from build123d import *

# Parameters (mm, degrees)
SKETCH_1_W          = 24
SKETCH_1_H          = 70
EXTRUDE_1_DEPTH     = 30
SKETCH_2_R          = 7.55
CUT_EXTRUDE_1_DEPTH = 71.806439045
SKETCH_3_W          = 25
SKETCH_3_H          = 10
CUT_EXTRUDE_2_DEPTH = 71.806439045
SKETCH_4_W          = 24
SKETCH_4_H          = 9.317438099
EXTRUDE_2_DEPTH     = 5
SKETCH_5_R          = 1.55
CUT_EXTRUDE_3_DEPTH = 31
FILLET_1_R          = 10


with BuildPart() as part:
    # 草图1 → 凸台-拉伸1 (new body)
    with BuildSketch(Plane(origin=(0, 0, 0), x_dir=(1, 0, 0), z_dir=(0, 1, 0))):
        with Locations((20.241900648, -24.477321814)):
            Rectangle(SKETCH_1_W, SKETCH_1_H)
    extrude(amount=EXTRUDE_1_DEPTH)

    # 草图2 → 切除-拉伸1 (cut, through all)
    with BuildSketch(Plane(origin=(32.241900648, 0, 0), x_dir=(0, 0, -1), z_dir=(1, 0, 0))):
        with Locations((-46.977321814, 15)):
            Circle(SKETCH_2_R)
        with Locations((-1.977321814, 15)):
            Circle(SKETCH_2_R)
    extrude(amount=-CUT_EXTRUDE_1_DEPTH, mode=Mode.SUBTRACT)

    # 草图3 → 切除-拉伸2 (cut, through all)
    with BuildSketch(Plane(origin=(32.241900648, 0, 0), x_dir=(0, 0, -1), z_dir=(1, 0, 0))):
        with Locations((-24.477321814, 15)):
            Rectangle(SKETCH_3_W, SKETCH_3_H)
    extrude(amount=-CUT_EXTRUDE_2_DEPTH, mode=Mode.SUBTRACT)

    # 草图4 → 凸台-拉伸2 (add)
    with BuildSketch(Plane(origin=(0, 30, 0), x_dir=(1, 0, 0), z_dir=(0, 1, 0))):
        with Locations((20.241900648, -17.269567559)):
            Rectangle(SKETCH_4_W, SKETCH_4_H)
    extrude(amount=EXTRUDE_2_DEPTH)

    # 草图5 → 切除-拉伸3 (cut)
    with BuildSketch(Plane(origin=(0, 35, 0), x_dir=(1, 0, 0), z_dir=(0, 1, 0))):
        with Locations(Location((27.441174565, -17.269567558, 0), (0, 0, 270))):
            Circle(SKETCH_5_R)
        with Locations(Location((13.141174565, -17.269567558, 0), (0, 0, 270))):
            Circle(SKETCH_5_R)
    extrude(amount=-CUT_EXTRUDE_3_DEPTH, mode=Mode.SUBTRACT)

    # 圆角1
    fillet_1_edges = [part.edges().sort_by_distance(p)[0] for p in [
        (20.241900648, 30, -10.522678186),
        (20.241900648, 0, -10.522678186),
        (20.241900648, 0, 59.477321814),
        (20.241900648, 30, 59.477321814),
    ]]
    fillet(fillet_1_edges, radius=FILLET_1_R)


solid = part.part
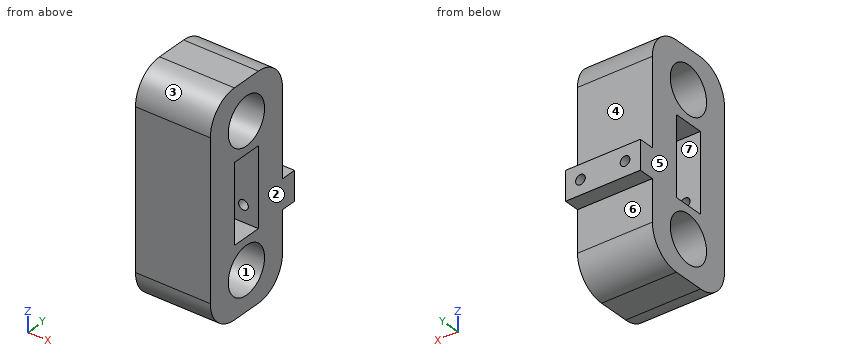
Design review of the part built by this model. Coordinates are the model's own, in mm. Face numbers are marked on the shaded views. A direction names the side the tool comes from. Round coordinates to 2 decimals unless told otherwise and drop trailing zeros. Loops run counter-clockwise (first coordinate to the right, second up) from the corner with the lowest first, then second, coordinate; pieces in that order, holes last. Notation, with made-up numbers: M 64.25,29 L 113.25,29 A20 ccw 113.25,65 Z; hole C 64.5,34 d4. An arc over 180 degrees is marked long. Answer as a JSON object with one key per item and string values.
Item 1: We need section A-A on y = 15. Give the boundary of the cut face in (x, z).
Answer sheet:
{"outline": "M 8.24,-10.52 L 32.24,-10.52 L 32.24,-5.57 L 8.24,-5.57 Z; M 8.24,9.53 L 32.24,9.53 L 32.24,11.98 L 8.24,11.98 Z; M 8.24,36.98 L 32.24,36.98 L 32.24,39.43 L 8.24,39.43 Z; M 8.24,54.53 L 32.24,54.53 L 32.24,59.48 L 8.24,59.48 Z"}
Item 2: We need section C-C on x = 18. Give the boundary of the cut face in (y, z).
Answer sheet:
{"outline": "M 0,-0.52 A10 ccw 10,-10.52 L 20,-10.52 A10 ccw 30,-0.52 L 30,12.61 L 35,12.61 L 35,21.93 L 30,21.93 L 30,49.48 A10 ccw 20,59.48 L 10,59.48 A10 ccw 0,49.48 Z; hole C 15,1.98 d15.1; hole C 15,46.98 d15.1; hole M 10,11.98 L 20,11.98 L 20,36.98 L 10,36.98 Z"}
Item 3: We need section D-D on z = 34.5. Give the boundary of the cut face in (x, y).
Answer sheet:
{"outline": "M 8.24,0 L 32.24,0 L 32.24,10 L 8.24,10 Z; M 8.24,20 L 32.24,20 L 32.24,30 L 8.24,30 Z"}
Item 4: The part is to be moulded in two halves that separate along Y. For the marked faces 1, 2, 3 and 4, say which applies: pulls with the +Y half, pulls with the -Y half, needs draft (parallel to the pull), parting line crosses it, or undercut.
Answer sheet:
{"face 1": "undercut", "face 2": "needs draft", "face 3": "pulls with the -Y half", "face 4": "pulls with the +Y half"}
Item 5: Machinability: for the marked faces 5, 6 and 7, which of the approach directions +Z, -Z, +X, -X, +Y, -Y give a long, thin tool a straight path to every point of the face, cutting with its end or side? Answer none if there is none.
Answer sheet:
{"face 5": "+Z, -Z, -X, +Y, -Y", "face 6": "-Z, +X, -X, +Y", "face 7": "+X, -X"}
Item 6: Clearance check with flat-ended pins moving along their axes: P1, Ø5, axis at x = 13.14, z = 17.27, coming from the +Y side; P2, Ø1.5, axis at x = 19, y = 22, coming from the -Z side; P3, Ø0.9, axis at x = 27, z = 16.5, coming from the +Y side; P4, Ø2, axis at x = 24, z = 44.5, coming from the +Y side. State where each tip first meets the part, or that it passes through.
Answer sheet:
{"P1": "stops at y = 35", "P2": "stops at z = -10.44", "P3": "stops at y = 4", "P4": "stops at y = 30"}
Item 7: We need section B-B on z = 20.5. Give the boundary of the cut face in (x, y).
Answer sheet:
{"outline": "M 8.24,0 L 32.24,0 L 32.24,10 L 8.24,10 Z; M 8.24,20 L 32.24,20 L 32.24,35 L 8.24,35 Z"}
Item 8: Wall thickness on L1, parallel to Y at x = 23.25, z = 16.5; L2, parallel to Z at x = 23.25, y = 18; L3, parallel to Y at x = 21.75, z = 47: over which ranges is each line inside the solid? List them lowest first. Write a range as from..to.
Answer sheet:
{"L1": "y = 0..10, 20..35", "L2": "z = -10.52..-4.95, 8.91..11.98, 36.98..40.05, 53.91..59.48", "L3": "y = 0..7.45, 22.55..30"}
